```python
from build123d import *

# Parameters (mm, degrees)
F0_R     = 3
F1_DEPTH = 3


with BuildPart() as f1:
    # F0 (on Front) → F1 (new body)
    with BuildSketch(Plane.XZ):
        with BuildLine():
            ThreePointArc((16, -8), (24, 0), (16, 8))
            Line((16, 8), (16, 16))
            Line((16, 16), (-4, 16))
            Line((-4, 16), (-4, 8))
            Line((-4, 8), (-16, 8))
            ThreePointArc((-16, 8), (-24, 0), (-16, -8))
            Line((-16, -8), (16, -8))
        make_face()
        with Locations((-16, 0)):
            Circle(F0_R, mode=Mode.SUBTRACT)
        with BuildLine():
            ThreePointArc((19, 0), (16, -3), (13, 0))
            ThreePointArc((13, 0), (13.8786796564, 2.1213203436), (16, 3))
            ThreePointArc((16, 3), (18.1213203436, 2.1213203436), (19, 0))
        make_face(mode=Mode.SUBTRACT)
    extrude(amount=F1_DEPTH)


solid = f1.part
```
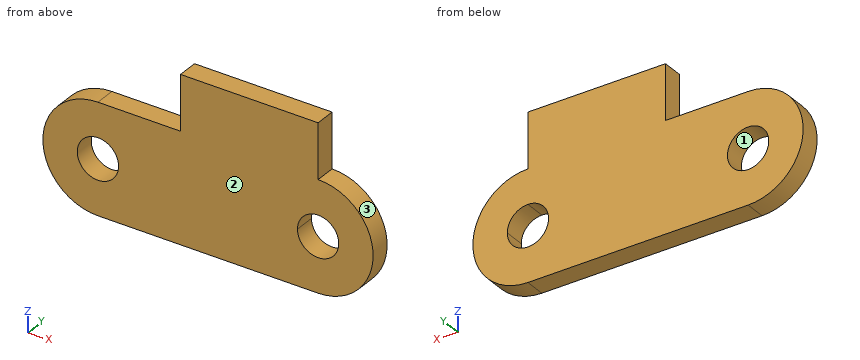
Check sheet for the modelled part. Datum: model origin and axes. Units: mm. Face numbers are marked on the shaded views. Give positions to 0.01 mm unless a question says otherwise; leave off trailing zeros. Order: outer loops, then holes, each group sorted by start corner. A loop starts at its lowest first (then second) coordinate and runs counter-clockwise, first axis right, second up. Notation, with made-up numbers: (16.25, 89.25) -> (22.25, 89.25) arc R9 ccw to (22.25, 99.25) -> close; hole circle Ø8 at (-7, 65.5). An arc over 180 degrees is marked (long way). Use CSV: the item, a comma, the result in double quotes. Start each with the question number.
1) Material ranges on line 1 (Z direction, x = -16, y = -0.85); line 2 (X direction, y = -0.3, z = 0.5); line 3 (Z direction, x = -4.5, y = -1.8), recorded low to high. Write a range as from..to.
2) Sectioned sample at B-B, the plane z = -1.75. Record the boundary of the cut face in (x, y), plus the area to 3 significant figures.
3) Sectioned sample at A-A, the plane y = -2.55. Record the boundary of the cut face in (x, z), plus the area to 3 significant figures.
4) Go/stop test with flat-tipped pins: P1, Ø0.9, axis at x = -11.5, y = -1, coming from the +Z side; P2, Ø1, axis at y = -1, z = -4, coming from the +X side; P3, Ø8, axis at x = 17.5, z = 9.5, coming from the +Y side; P4, Ø1.5, axis at y = -0.5, z = -2.5, coming from the +X side. Record where each tip stops, or that it passes through.
5) Mould release check, pull along X, two halves, no side actions. Record for the marked faces 1, 2 and 3: released by +X, released by -X, zero draft, split by the parting line, or undercut.
6) Sectioned sample at D-D, the plane x = -5.5. Record the boundary of the cut face in (y, z), plus the area to 3 significant figures.
7) Sectioned sample at C-C, the plane x = 15. Record the boundary of the cut face in (y, z), plus the area to 3 significant figures.
Recorded:
1,line 1,"-8..-3, 3..8"
1,line 2,"-23.98..-18.96, -13.04..13.04, 18.96..23.98"
1,line 3,"-8..8"
2,outline,"(-23.81, -3) -> (-18.44, -3) -> (-18.44, 0) -> (-23.81, 0) -> close; (-13.56, -3) -> (13.56, -3) -> (13.56, 0) -> (-13.56, 0) -> close; (18.44, -3) -> (23.81, -3) -> (23.81, 0) -> (18.44, 0) -> close"
2,area,"114 mm2"
3,outline,"(-16, -8) -> (16, -8) arc R8 ccw to (16, 8) -> (16, 16) -> (-4, 16) -> (-4, 8) -> (-16, 8) arc R8 ccw to start; hole circle Ø6 at (-16, 0); hole circle Ø6 at (16, 0)"
3,area,"817 mm2"
4,P1,"z = 8"
4,P2,"x = 23.19"
4,P3,"y = 0"
4,P4,"x = 23.81"
5,face 1,"undercut"
5,face 2,"zero draft"
5,face 3,"released by +X"
6,outline,"(-3, -8) -> (0, -8) -> (0, 8) -> (-3, 8) -> close"
6,area,"48.0 mm2"
7,outline,"(-3, -8) -> (0, -8) -> (0, -2.83) -> (-3, -2.83) -> close; (-3, 2.83) -> (0, 2.83) -> (0, 16) -> (-3, 16) -> close"
7,area,"55.0 mm2"
